```python
from build123d import *

# Parameters (mm, degrees)
F0_W     = 89.916
F0_H     = 59.436
F0_W_2   = 83.82
F0_H_2   = 53.34
F1_DEPTH = 3.048
F2_DEPTH = 20.828
F3_R     = 2.54


with BuildPart() as f1:
    # F0 (on Top) → F1 (new body)
    with BuildSketch(Plane.XY):
        with Locations((-44.958, 29.718)):
            Rectangle(F0_W, F0_H)
        with Locations((-44.958, 29.718)):
            Rectangle(F0_W_2, F0_H_2, mode=Mode.SUBTRACT)
        with Locations((-44.958, 29.718)):
            Rectangle(F0_W_2, F0_H_2)
    extrude(amount=-F1_DEPTH)

    # F0 (on Top) → F2 (join)
    with BuildSketch(Plane.XY):
        with Locations((-44.958, 29.718)):
            Rectangle(F0_W, F0_H)
        with Locations((-44.958, 29.718)):
            Rectangle(F0_W_2, F0_H_2, mode=Mode.SUBTRACT)
    extrude(amount=F2_DEPTH)

    # F3
    f3_edges = [f1.edges().sort_by_distance(p)[0] for p in [
        (0, 0, 8.89),
        (0, 59.436, 8.89),
        (-89.916, 59.436, 8.89),
        (-89.916, 0, 8.89),
    ]]
    fillet(f3_edges, radius=F3_R)


solid = f1.part
```
Build history of the part. All positions in model axes, mm. A direction names the side the tool comes from. Give positions to 0.01 mm unless a question says otherwise; leave off trailing zeros. Loops run counter-clockwise (first coordinate to the right, second up) from the corner with the lowest first, then second, coordinate; pieces in that order, holes last. Notation, with made-up numbers: (-12.5, -3.75) -> (31.5, -3.75) arc R17 cw to (31.5, 11.25) -> close; hole circle Ø11 at (15, 87). An arc over 180 degrees is marked (long way). One line per question, with ' | ' between items. Start each with the question number.
1) Pin check, flat tip, straight feed: pin 1 (3 mm diameter, centred on x = -52.5, y = 44.5, fed in from +Z). Stop position of the tip, or through.
2) Two-plate mould, pull along X, no slides. Class faces 3 (the flat face through (-46, 0, 9)), 4 (the flat face through (-86.868, 29, 10)), 5 (the cylindrical face through (-0.72, 58.67, 8.72)): released by +X, released by -X, zero draft, split by the parting line, or undercut.
3) 3-axis set-ups, long thin cutter, end or side, ignore diameter. For faces 1 (the cylindrical face through (-0.764, 0.724, 9.057)), 2 (the flat face through (-46, 56.388, 10)): which of +Z, -Z, +X, -X, +Y, -Y reach the whole face in a straight line?
4) Cut at B-B (y = 36). Give the cut face in (x, z).
5) Cut at C-C (x = -70.5). Give the cut face in (y, z).
6) Probe L1, parallel to X at y = 19.5, z = 0.75; L2, parallel to Y at x = -12, z = 17.5; L3, parallel to Z at x = -44, y = 11.5. List the from-to ranges inside material, lowest first.
7) Cut at A-A (z = 14.75). Give the cut face in (x, y).
Return value:
1) pin 1: z = 0
2) face 3: zero draft | face 4: undercut | face 5: released by +X
3) face 1: +Z, -Z, +X, -Y | face 2: +Z
4) outline: (-89.92, -3.05) -> (0, -3.05) -> (0, 20.83) -> (-3.05, 20.83) -> (-3.05, 0) -> (-86.87, 0) -> (-86.87, 20.83) -> (-89.92, 20.83) -> close
5) outline: (0, -3.05) -> (59.44, -3.05) -> (59.44, 20.83) -> (56.39, 20.83) -> (56.39, 0) -> (3.05, 0) -> (3.05, 20.83) -> (0, 20.83) -> close
6) L1: -89.92 to -86.87, -3.05 to 0 | L2: 0 to 3.05, 56.39 to 59.44 | L3: -3.05 to 0
7) outline: (-89.92, 2.54) arc R2.54 ccw to (-87.38, 0) -> (-2.54, 0) arc R2.54 ccw to (0, 2.54) -> (0, 56.9) arc R2.54 ccw to (-2.54, 59.44) -> (-87.38, 59.44) arc R2.54 ccw to (-89.92, 56.9) -> close; hole (-86.87, 3.05) -> (-3.05, 3.05) -> (-3.05, 56.39) -> (-86.87, 56.39) -> close
